```python
from build123d import *

# Parameters (mm, degrees)
BOSS_EXTRUDE1_DEPTH = 13.5
SKETCH2_R           = 1.5
CUT_EXTRUDE1_DEPTH  = 20
CUT_EXTRUDE2_DEPTH  = 3.5


with BuildPart() as part:
    # Sketch1 → Boss-Extrude1 (new body, symmetric)
    with BuildSketch(Plane(origin=(0, 0, 0), x_dir=(0, 0, -1), z_dir=(1, 0, 0))):
        Polygon((0, 0), (-12, 0), (-12, 3), (-2.5, 3), (-2.5, 20), (0, 20), align=None)
    extrude(amount=BOSS_EXTRUDE1_DEPTH, both=True)

    # Sketch2 → Cut-Extrude1 (cut)
    with BuildSketch(Plane(origin=(0, 3, 0), x_dir=(1, 0, 0), z_dir=(0, 1, 0))):
        with Locations((-9, -6)):
            Circle(SKETCH2_R)
        with Locations((9, -6)):
            Circle(SKETCH2_R)
    extrude(amount=-CUT_EXTRUDE1_DEPTH, mode=Mode.SUBTRACT)

    # Sketch3 → Cut-Extrude2 (cut, through all)
    with BuildSketch(Plane.XY.offset(2.5)):
        with BuildLine():
            Line((-6.000505089, 15.5), (-6.000505089, 7))
            ThreePointArc((-6.000505089, 7), (-7.5, 5.500505089), (-8.999494911, 7))
            Line((-8.999494911, 7), (-8.999494911, 15.5))
            ThreePointArc((-8.999494911, 15.5), (-7.5, 16.999494911), (-6.000505089, 15.5))
        make_face()
        with BuildLine():
            Line((8.999494911, 15.5), (8.999494911, 7))
            ThreePointArc((8.999494911, 7), (7.5, 5.500505089), (6.000505089, 7))
            Line((6.000505089, 7), (6.000505089, 15.5))
            ThreePointArc((6.000505089, 15.5), (7.5, 16.999494911), (8.999494911, 15.5))
        make_face()
    extrude(amount=-CUT_EXTRUDE2_DEPTH, mode=Mode.SUBTRACT)


solid = part.part
```
Read the model definition and answer for the solid it produces. Units are mm, in the model's axes. A direction names the side the tool comes from. Coordinates: 2 decimals unless noted, no trailing zeros. Loops run counter-clockwise (first coordinate to the right, second up) from the corner with the lowest first, then second, coordinate; pieces in that order, holes last.
(1) The mould has two halves that part along Z. Classify faces 4 (the face through (7.8, 1.5, 6.9)), 5 (the face through (0, 11, 2.5)), 6 (the face through (-7.5, 5.5, 1.3)): released by +Z, released by -Z, zero draft, split by the parting line, or undercut.
Solution:
face 4: undercut
face 5: released by +Z
face 6: zero draft
(2) The part is cut by section C-C (x = 4.5). Determine the outline of the cut face in (y, z).
Solution:
outline: (0, 0) - (20, 0) - (20, 2.5) - (3, 2.5) - (3, 12) - (0, 12) - close
(3) The part is cut by section D-D (z = 2). Determine the outline of the cut face in (x, y).
Solution:
outline: (-13.5, 0) - (13.5, 0) - (13.5, 20) - (-13.5, 20) - close; hole (-9, 7) arc R1.5 ccw to (-6, 7) - (-6, 15.5) arc R1.5 ccw to (-9, 15.5) - close; hole (6, 7) arc R1.5 ccw to (9, 7) - (9, 15.5) arc R1.5 ccw to (6, 15.5) - close
(4) A tool of negligible diameter and unlimited length cuts with its end or side. For faces 1 (the face through (0, 1, 12)), 2 (the face through (0, 3, 7)), 3 (the face through (8.999, 11, 1)), from which of +Z, -Z, +X, -X, +Y, -Y can it reach the whole face along a straight path? Write none if from no direction.
Solution:
face 1: +Z, +X, -X, +Y, -Y
face 2: +Z, +X, -X, +Y
face 3: +Z, -Z
(5) The part is cut by section A-A (z = 6). Determine the outline of the cut face in (x, y).
Solution:
outline: (-13.5, 0) - (-10.5, 0) - (-10.5, 3) - (-13.5, 3) - close; (-7.5, 0) - (7.5, 0) - (7.5, 3) - (-7.5, 3) - close; (10.5, 0) - (13.5, 0) - (13.5, 3) - (10.5, 3) - close
(6) Flat-ended cylindrical pins translate along their axes: pin 1 Ø1.5 at (x, y) = (3.5, 18) entering from +Z; pin 2 Ø5 at (x, z) = (-9, 6) entering from +Y. Find the tip coordinate at first contact, or state that the pin passes through.
Solution:
pin 1: stops at z = 2.5
pin 2: stops at y = 3
(7) The part is cut by section B-B (y = 12). Determine the outline of the cut face in (x, z), and give its area (3 significant figures).
Solution:
outline: (-13.5, 0) - (-9, 0) - (-9, 2.5) - (-13.5, 2.5) - close; (-6, 0) - (6, 0) - (6, 2.5) - (-6, 2.5) - close; (9, 0) - (13.5, 0) - (13.5, 2.5) - (9, 2.5) - close
area: 52.5 mm2
(8) Consider line 1 along X through (y, z) = (14, 1.25); line 2 along X through (y, z) = (2.45, 6); line 3 along Z through (x, y) = (-9, 1.55). Determine where each line is inside the solid, lowest interval first.
Solution:
line 1: x = -13.5 to -9, -6 to 6, 9 to 13.5
line 2: x = -13.5 to -10.5, -7.5 to 7.5, 10.5 to 13.5
line 3: z = 0 to 4.5, 7.5 to 12
